For this review, take the finished solid that the model builds, in its own axes (mm). Face numbers are marked on the shaded views. A direction names the side the tool comes from. Round coordinates to 2 decimals unless told otherwise and drop trailing zeros. Order: outer loops, then holes, each group sorted by start corner. A loop starts at its lowest first (then second) coordinate and runs counter-clockwise, first axis right, second up. Notation, with made-up numbers: M 17.5,52 L 41.5,52 A23 ccw 41.5,90 Z; hole C -2.75,87 d1. An arc over 180 degrees is marked long. Use a Markdown table: item, result.
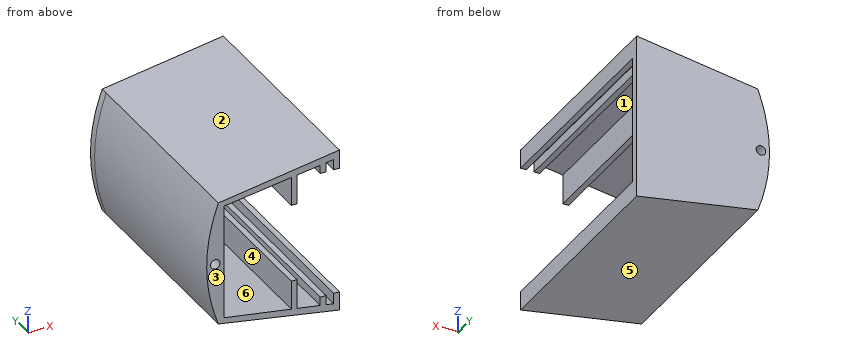
from build123d import *

# Parameters (mm, degrees)
SALIENTE_EXTRUIR11_DEPTH   = 110
SALIENTE_EXTRUIR12_DEPTH   = 4
CROQUIS7_R                 = 2.5
CORTAR_EXTRUIR2_DEPTH      = 1.0000001
CORTAR_EXTRUIR2_DEPTH_BACK = 115.0000001


with BuildPart() as part:
    # Croquis1 → Saliente-Extruir11 (new body)
    with BuildSketch(Plane(origin=(0, 0, 0), x_dir=(1, 0, 0), z_dir=(0, 1, 0))):
        with BuildLine():
            Line((27.20407189, 42.896490362), (27.20407189, 39.115188491))
            Line((27.20407189, 39.115188491), (27.20407189, 33.115188491))
            Line((27.20407189, 33.115188491), (24.20407189, 33.115188491))
            Line((24.20407189, 33.115188491), (24.20407189, 38.659429067))
            Line((24.20407189, 38.659429067), (20.20407189, 38.051749834))
            Line((20.20407189, 38.051749834), (20.20407189, 33.115188491))
            Line((20.20407189, 33.115188491), (17.20407189, 33.115188491))
            Line((17.20407189, 33.115188491), (17.20407189, 37.59599041))
            Line((17.20407189, 37.59599041), (5.20407189, 35.772952711))
            Line((5.20407189, 35.772952711), (5.20407189, 20.317193287))
            Line((5.20407189, 20.317193287), (2.20407189, 20.317193287))
            Line((2.20407189, 20.317193287), (2.20407189, 35.317193287))
            Line((2.20407189, 35.317193287), (-32.79592811, 30))
            Line((-32.79592811, 30), (-32.79592811, -30))
            Line((-32.79592811, -30), (2.20407189, -35.428420748))
            Line((2.20407189, -35.428420748), (2.20407189, -20.428420748))
            Line((2.20407189, -20.428420748), (5.20407189, -20.428420748))
            Line((5.20407189, -20.428420748), (5.20407189, -35.893713955))
            Line((5.20407189, -35.893713955), (17.20407189, -37.754886783))
            Line((17.20407189, -37.754886783), (17.20407189, -33.30586414))
            Line((17.20407189, -33.30586414), (20.20407189, -33.30586414))
            Line((20.20407189, -33.30586414), (20.20407189, -38.22017999))
            Line((20.20407189, -38.22017999), (24.20407189, -38.840570933))
            Line((24.20407189, -38.840570933), (24.20407189, -33.30586414))
            Line((24.20407189, -33.30586414), (27.20407189, -33.30586414))
            Line((27.20407189, -33.30586414), (27.20407189, -39.30586414))
            Line((27.20407189, -39.30586414), (27.20407189, -43.103509638))
            Line((27.20407189, -43.103509638), (-35.710171222, -32.509265277))
            add(Edge.make_bspline(
                [(-35.745382219, 32.513512597), (-47.864078296, -0.004370105), (-35.710171222, -32.509265277)],
                knots=[0, 0, 0, 1, 1, 1], degree=2))
            Line((-35.745382219, 32.513512597), (27.20407189, 42.896490362))
        make_face()
    extrude(amount=SALIENTE_EXTRUIR11_DEPTH)

    # Croquis6 → Saliente-Extruir12 (add)
    with BuildSketch(Plane(origin=(0, 110, 0), x_dir=(1, 0, 0), z_dir=(0, 1, 0))):
        with BuildLine():
            Line((-35.745382219, 32.513512597), (27.20407189, 42.896490362))
            Line((27.20407189, 42.896490362), (27.20407189, -43.103509638))
            Line((27.20407189, -43.103509638), (-35.710171222, -32.509265277))
            add(Edge.make_bspline(
                [(-35.745382219, 32.513512597), (-47.864078276, -0.004407917), (-35.710171222, -32.509265277)],
                knots=[0, 0, 0, 1, 1, 1], degree=2))
        make_face()
    extrude(amount=SALIENTE_EXTRUIR12_DEPTH)

    # Croquis7 → Cortar-Extruir2 (cut, two sides)
    with BuildSketch(Plane.XZ) as cortar_extruir2_sk:
        with Locations((-37.356797981, 0)):
            Circle(CROQUIS7_R)
    extrude(amount=CORTAR_EXTRUIR2_DEPTH, mode=Mode.SUBTRACT)
    extrude(cortar_extruir2_sk.sketch, amount=-CORTAR_EXTRUIR2_DEPTH_BACK, mode=Mode.SUBTRACT)


solid = part.part
Q1. Wall thickness on line 1 along Y through (x, z) = (14.5, -19); line 2 along X through (y, z) = (76.5, -29); line 3 along Z through (x, y) = (-13, 60.5): over which ranges is each line inside the solid? List them lowest first. Write a range as [from, to].
Determined:
| item | result |
|---|---|
| line 1 | y = [110, 114] |
| line 2 | x = [-36.98, -32.8], [2.2, 5.2] |
| line 3 | z = [-36.27, -33.01], [33.07, 36.33] |
Q2. Clearance check with flat-ended pins moving along their axes: pin 1 (12 mm diameter, centred on y = 58, z = -26.5, fed in from -X); pin 2 (4.5 mm diameter, centred on y = 30.5, z = 26.5, fed in from -X); pin 3 (1.5 mm diameter, centred on x = 4, y = 31, fed in from +Z). State where each tip first meets the part, or that it passes through.
Determined:
| item | result |
|---|---|
| pin 1 | stops at x = -39.39 |
| pin 2 | stops at x = -38.41 |
| pin 3 | stops at z = 39.32 |
Q3. Machinability: for the marked faces 5 and 6, which of the approach directions +Z, -Z, +X, -X, +Y, -Y give a long, thin tool a straight path to every point of the face, cutting with its end or side? Answer none if there is none.
Determined:
| item | result |
|---|---|
| face 5 | -Z, -X, +Y, -Y |
| face 6 | -Y |
Q4. Add section A-A (x = -17). Write out the cut boundary in (y, z).
Determined:
| item | result |
|---|---|
| outline | M 0,-35.61 L 114,-35.61 L 114,35.66 L 0,35.66 L 0,32.45 L 110,32.45 L 110,-32.4 L 0,-32.4 Z |
Q5. Draft analysis for pull direction X (two halves, no side actions). For the marked faces 1, 2, 3 and 4, state which applies: pulls with the +X half, pulls with the -X half, needs draft (parallel to the pull), parting line crosses it, or undercut.
Determined:
| item | result |
|---|---|
| face 1 | undercut |
| face 2 | pulls with the -X half |
| face 3 | needs draft |
| face 4 | undercut |
Q6. Add section B-B (x = -27). Write out the cut boundary in (y, z), then the cut area to 3 significant figures.
Determined:
| item | result |
|---|---|
| outline | M 0,-33.96 L 114,-33.96 L 114,33.98 L 0,33.98 L 0,30.9 L 110,30.9 L 110,-30.88 L 0,-30.88 Z |
| area | 949 mm^2 |
